Can you work these out from the model? Positions are in its coordinate system, mm. Face numbers are marked on the shaded views. A direction names the side the tool comes from. Give positions to 0.01 mm unless a question says otherwise; leave off trailing zeros. Order: outer loops, then holes, each group sorted by start corner. A loop starts at its lowest first (then second) coordinate and runs counter-clockwise, first axis right, second up.
Item 1: I want a section at A-A, the plane z = 0. Write out the boundary of the cut face in (x, y), then the cut area to 3 significant figures.
Item 2: I'm going to push flat-ended pins straight in: pin 1 Ø8 at (x, y) = (58.5, 13) entering from -Z; pin 2 Ø8 at (x, y) = (84, 1.5) entering from +Z; pin 3 Ø12 at (x, z) = (50.5, 10.5) entering from +Y. Where does each tip first touch, or does it pass through?
Item 3: I want a section at D-D, the plane x = 113. Write out the boundary of the cut face in (y, z), then the cut area to 3 significant figures.
Item 4: If I drill on line 1 along Z through (x, y) = (73, 1); line 2 along X through (y, z) = (-14.5, -15); line 3 along Z through (x, y) = (112, 1), over which ranges is the centre line in solid material (lowest first)?
Item 5: Which directions (+Z, -Z, +X, -X, +Y, -Y) give clear straight access to the entire face, cutting with the end or side of a thin tool? Please do the marked faces 1, 2 and 3.
Item 6: I want a section at C-C, the plane x = 47. Write out the boundary of the cut face in (y, z).
Autodesk Inventor part; units mm, degrees
ref_plane "Start Plane" through (0, 0, 0) normal (1, 0, 0) x (0, 1, 0)
ref_plane "XZ Plane" through (0, 0, 0) normal (0, 1, 0) x (-1, 0, 0)
ref_plane "XY Plane" through (0, 0, 0) normal (0, 0, 1) x (1, 0, 0)
sketch "Main Sketch" plane through (0, 0, 0) normal (0, 0, 1) x (1, 0, 0)
  line L0 (0, 0) -> (209.5, 0)
  line L1 (0, 0) -> (0, 17.5)
  line L2 (0, 17.5) -> (40, 17.5)
  line L3 (40, 17.5) -> (40, 22.5)
  line L4 (45, 22.5) -> (45, 20)
  line L5 (40, 22.5) -> (45, 22.5)
  line L6 (103, 20) -> (103, 17.75)
  line L7 (45, 20) -> (103, 20)
  line L8 (139.5, 17.75) -> (139.5, 17.5)
  line L9 (103, 17.75) -> (139.5, 17.75)
  line L10 (179.5, 17.5) -> (179.5, 15.25)
  line L11 (139.5, 17.5) -> (179.5, 17.5)
  line L12 (209.5, 15.25) -> (209.5, 0)
  line L13 (179.5, 15.25) -> (209.5, 15.25)
  dimension "d3" = 35
  dimension "d4" = 45
  dimension "d5" = 40
  dimension "d6" = 35.5
  dimension "d7" = 35
  dimension "d8" = 30.5
revolve "Revolution1" add sketch "Main Sketch" angle 360 about axis through (0, 0, 0) along (1, 0, 0)
chamfer "Chamfer1" distance 2 angle 45 1 edges at (0, -17.5, 0) measured on face at (26.6667, 17.4433, -1.4082)
chamfer "Chamfer2" distance 2 angle 45 1 edges at (209.5, -15.25, 0) measured on face at (199.5, 15.2005, -1.2271)
equation "\"Length\" = 209.5"
properties part number "Shaft" material "Steel"
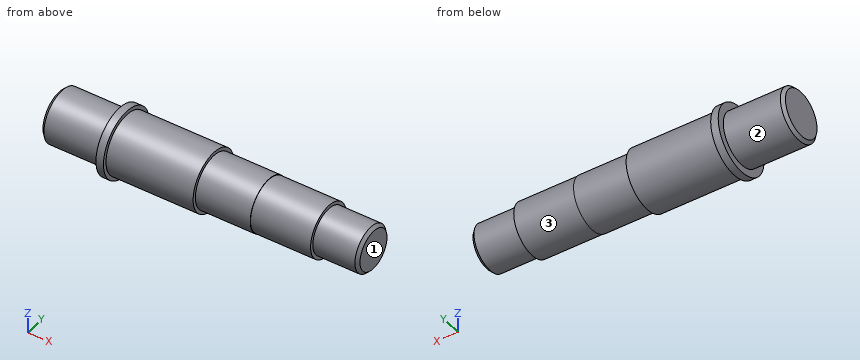
Results list:
1. outline: (0, -15.5) - (2, -17.5) - (40, -17.5) - (40, -22.5) - (45, -22.5) - (45, -20) - (103, -20) - (103, -17.75) - (139.5, -17.75) - (139.5, -17.5) - (179.5, -17.5) - (179.5, -15.25) - (207.5, -15.25) - (209.5, -13.25) - (209.5, 13.25) - (207.5, 15.25) - (179.5, 15.25) - (179.5, 17.5) - (139.5, 17.5) - (139.5, 17.75) - (103, 17.75) - (103, 20) - (45, 20) - (45, 22.5) - (40, 22.5) - (40, 17.5) - (2, 17.5) - (0, 15.5) - close
1. area: 7,550 mm2
2. pin 1: stops at z = -17.86
2. pin 2: stops at z = 20
2. pin 3: stops at y = 20.99
3. outline: circle Ø35.5 at (0, 0)
3. area: 990 mm2
4. line 1: z = -19.97 to 19.97
4. line 2: x = 40 to 45
4. line 3: z = -17.72 to 17.72
5. face 1: +Z, -Z, +X, +Y, -Y
5. face 2: -X
5. face 3: +X
6. outline: circle Ø40 at (0, 0)
